CAD build for the part. Positions are in the model's coordinates, mm. Round coordinates to 2 decimals unless told otherwise and drop trailing zeros. Write each loop counter-clockwise with the first axis right and the second up, starting at its lowest first coordinate (ties: lowest second). Pieces come first, ordered by that corner, then holes. Notation, with made-up numbers: (-31.5, 60.5) -> (23.5, 60.5) arc R13 ccw to (23.5, 74.5) -> close; hole circle Ø6 at (39.25, 53). An arc over 180 degrees is marked (long way). Put each result on its own line as item: value. Start each with the question number.
1. Drill centre lines: line 1 (Z direction, x = 118, y = 0); line 2 (Z direction, x = 7, y = 4.75); line 3 (Y direction, x = 80, z = -3.75). Where is each one in solid material? Low to high. Write a range as from..to.
2. Saw through at A-A on z = 0. List the corners of the cut face in (x, y), and give its area (3 significant figures).
3. Flat gauge pins, fed straight in: P1, Ø1, axis at x = 68, y = -3, coming from the -Z side; P2, Ø0.7, axis at x = 50, y = -4, coming from the -Z side; P3, Ø1, axis at x = 130.5, y = 1.5, coming from the -Z side. Where does each tip first touch, or does it go through?
Autodesk Inventor part; units mm, degrees
ref_plane "YZ Plane" through (0, 0, 0) normal (1, 0, 0) x (0, 1, 0)
ref_plane "XZ Plane" through (0, 0, 0) normal (0, 1, 0) x (-1, 0, 0)
ref_plane "XY Plane" through (0, 0, 0) normal (0, 0, 1) x (1, 0, 0)
sketch "Sketch1" plane through (0, 0, 0) normal (1, 0, 0) x (0, 1, 0)
  line L0 (-10, -10) -> (10, -10)
  line L1 (10, -10) -> (10, 10)
  line L2 (10, 10) -> (-10, 10)
  line L3 (-10, 10) -> (-10, -10)
  line L4 (-10, -10) -> (10, 10) construction
  line L5 (10, -10) -> (-10, 10) construction
  line L6 (10, 4.9) -> (8.2, 3.1)
  line L7 (8.2, 3.1) -> (8.2, 5.4993)
  line L8 (8.2, 5.4993) -> (6.56, 5.4993)
  line L9 (6.56, 5.4993) -> (3.9007, 2.84)
  line L10 (3.9007, -2.84) -> (6.56, -5.4993)
  line L11 (6.56, -5.4993) -> (8.2, -5.4993)
  line L12 (8.2, -5.4993) -> (8.2, -3.1)
  line L13 (8.2, -3.1) -> (10, -4.9)
  circle A0 centre (0, 0) radius 2.4
  line L14 (3.9007, 2.84) -> (3.9007, -2.84)
  line L15 (3.9007, 0) -> (0, 0) construction
  line L16 (5.4993, 6.56) -> (5.4993, 8.2)
  line L17 (2.84, 3.9007) -> (5.4993, 6.56)
  line L18 (-2.84, 3.9007) -> (2.84, 3.9007)
  line L19 (-5.4993, 6.56) -> (-2.84, 3.9007)
  line L20 (-5.4993, 8.2) -> (-5.4993, 6.56)
  line L21 (-3.1, 8.2) -> (-5.4993, 8.2)
  line L22 (-4.9, 10) -> (-3.1, 8.2)
  line L23 (3.1, 8.2) -> (4.9, 10)
  line L24 (5.4993, 8.2) -> (3.1, 8.2)
  line L25 (-6.56, 5.4993) -> (-8.2, 5.4993)
  line L26 (-3.9007, 2.84) -> (-6.56, 5.4993)
  line L27 (-3.9007, -2.84) -> (-3.9007, 2.84)
  line L28 (-6.56, -5.4993) -> (-3.9007, -2.84)
  line L29 (-8.2, -5.4993) -> (-6.56, -5.4993)
  line L30 (-8.2, -3.1) -> (-8.2, -5.4993)
  line L31 (-10, -4.9) -> (-8.2, -3.1)
  line L32 (-8.2, 3.1) -> (-10, 4.9)
  line L33 (-8.2, 5.4993) -> (-8.2, 3.1)
  line L34 (-5.4993, -6.56) -> (-5.4993, -8.2)
  line L35 (-2.84, -3.9007) -> (-5.4993, -6.56)
  line L36 (2.84, -3.9007) -> (-2.84, -3.9007)
  line L37 (5.4993, -6.56) -> (2.84, -3.9007)
  line L38 (5.4993, -8.2) -> (5.4993, -6.56)
  line L39 (3.1, -8.2) -> (5.4993, -8.2)
  line L40 (4.9, -10) -> (3.1, -8.2)
  line L41 (-3.1, -8.2) -> (-4.9, -10)
  line L42 (-5.4993, -8.2) -> (-3.1, -8.2)
  point P0 (0, 3.9007)
  point P1 (-3.9007, 0)
  point P2 (0, -3.9007)
  dimension "d0" = 20
  dimension "d1" = 20
  dimension "d2" = 45
  dimension "d3" = 45
  dimension "d4" = 1.8
  dimension "d5" = 1.8
  dimension "d6" = 4.8
  dimension "d7" = 1.64
  dimension "d8" = 1.64
  dimension "d11" = 5.68
  dimension "d12" = 3.1
  dimension "d13" = 3.1
  dimension "d16" = 360
  dimension "d18" = 1.5
  dimension "d19" = 2.3993
  dimension "d20" = 2.3993
extrude "Extrusion1" add sketch "Sketch1" along normal blind 150 contours L3 L31 L30 L29 L28 L27 L26 L25 L33 L32 L2 L22 L21 L20 L19 L18 L17 L16 L24 L23 L1 L6 L7 L8 L9 L14 L10 L11 L12 L13 L0 L40 L39 L38 L37 L36 L35 L34 L42 L41
equation "\"d3\" = d2"
equation "\"d5\" = d4"
equation "\"d8\" = d7"
equation "\"d19\" = d20"
properties part number "2020" material "Aluminum 6061"
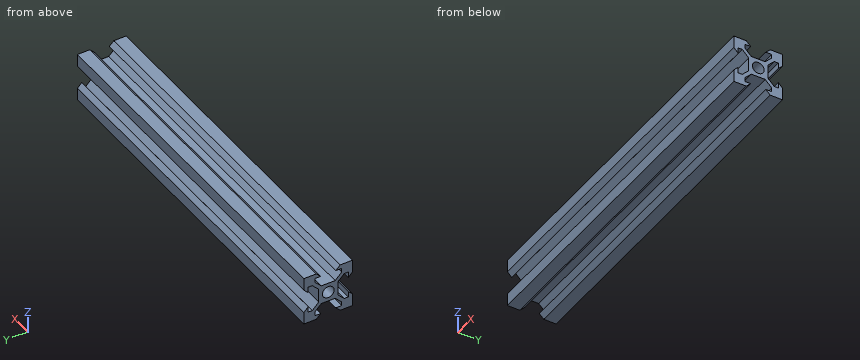
Return value:
1. line 1: z = -3.9..-2.4, 2.4..3.9
1. line 2: z = -9.85..-8.2, -5.81..-3.69, 3.69..5.81, 8.2..9.85
1. line 3: y = -8.85..-8.2, -4.81..4.81, 8.2..8.85
2. outline: (0, -3.9) -> (150, -3.9) -> (150, -2.4) -> (0, -2.4) -> close; (0, 2.4) -> (150, 2.4) -> (150, 3.9) -> (0, 3.9) -> close
2. area: 450 mm^2
3. P1: stops at z = -8.6
3. P2: stops at z = -9.45
3. P3: stops at z = -3.9
